Source: CAD feature listing. Evaluate the final solid. Frame: model axes, mm. Coordinates: 2 decimals unless noted, no trailing zeros. Loops run counter-clockwise (first coordinate to the right, second up) from the corner with the lowest first, then second, coordinate; pieces in that order, holes last. Notation, with made-up numbers: (13, 78.5) -> (22, 78.5) arc R19 cw to (22, 102.5) -> close; hole circle Ø2 at (-10.5, 59.5). An arc over 180 degrees is marked (long way). Answer as a JSON object with one key per item and string values. Group by question number.
from build123d import *

# Parameters (mm, degrees)
PLAT_W                          = 30
PLAT_H                          = 5
EL_MENT_M_CANO_SOUD_1_DEPTH     = 812
DIAM_TRE_DU_PER_AGE_13_0_13_1_D = 13
R_P_TITION_LIN_AIRE2_COUNT      = 3
R_P_TITION_LIN_AIRE2_PITCH      = 376


with BuildPart() as part:
    # plat → Elément mécano-soudé1 (new body)
    with BuildSketch(Plane.YZ.offset(-406)):
        Rectangle(PLAT_W, PLAT_H)
    extrude(amount=EL_MENT_M_CANO_SOUD_1_DEPTH)

    # Diamètre du perçage Ø13.0 (13)1 (through all)
    with Locations(Plane(origin=(0, 0, -2.5), x_dir=(-1, 0, 0), z_dir=(0, 0, -1))):
        with Locations((376, 0)):
            diam_tre_du_per_age_13_0_13_1 = Hole(DIAM_TRE_DU_PER_AGE_13_0_13_1_D / 2)

    # Répétition linéaire2: Diamètre du perçage Ø13.0 (13)1 ×3
    with Locations(*[(i * R_P_TITION_LIN_AIRE2_PITCH, 0, 0) for i in range(1, R_P_TITION_LIN_AIRE2_COUNT)]):
        add(diam_tre_du_per_age_13_0_13_1, mode=Mode.SUBTRACT)


solid = part.part
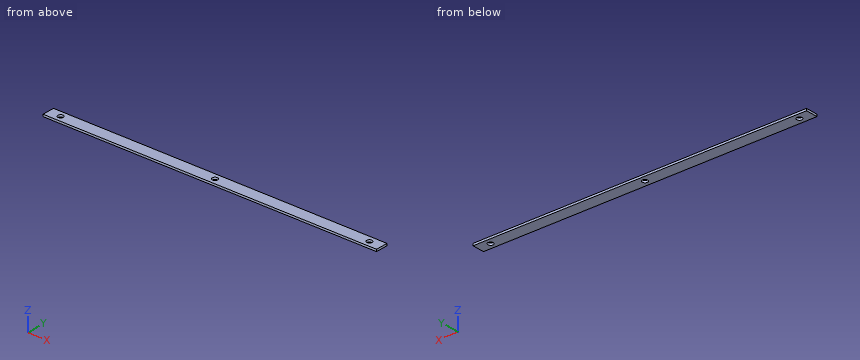
1. Section query B-B on z = 0.95. Return loops of the section in (x, y).
2. Ray query, L1, parallel to Y at x = 376, z = -0.05; L2, parallel to X at y = -2.75, z = -2.05; L3, parallel to X at y = -2.25, z = -2.3. Return the intervals inside material, ascending.
3. Section query A-A on y = 0. Return loops of the section in (x, z).
Solved:
{
 "1": {"outline": "(-406, -15) -> (406, -15) -> (406, 15) -> (-406, 15) -> close; hole circle Ø13 at (-376, 0); hole circle Ø13 at (0, 0); hole circle Ø13 at (376, 0)"},
 "2": {"L1": "-15 to -6.5, 6.5 to 15", "L2": "-406 to -381.89, -370.11 to -5.89, 5.89 to 370.11, 381.89 to 406", "L3": "-406 to -382.1, -369.9 to -6.1, 6.1 to 369.9, 382.1 to 406"},
 "3": {"outline": "(-406, -2.5) -> (-382.5, -2.5) -> (-382.5, 2.5) -> (-406, 2.5) -> close; (-369.5, -2.5) -> (-6.5, -2.5) -> (-6.5, 2.5) -> (-369.5, 2.5) -> close; (6.5, -2.5) -> (369.5, -2.5) -> (369.5, 2.5) -> (6.5, 2.5) -> close; (382.5, -2.5) -> (406, -2.5) -> (406, 2.5) -> (382.5, 2.5) -> close"}
}
